Verification items for this drawing (mm, ordinates from the low corner). A direction names the side the tool comes from. Round coordinates to 2 decimals unless told otherwise and drop trailing zeros. Order: outer loops, then holes, each group sorted by start corner. A loop starts at its lowest first (then second) coordinate and runs counter-clockwise, first axis right, second up. Notation, with made-up numbers: (47, 22.25) -> (84, 22.25) arc R7 ccw to (84, 26.25) -> close; hole circle Ø3 at (-32, 67.5). An arc over 180 degrees is marked (long way). Put each result on its own line as item: value.
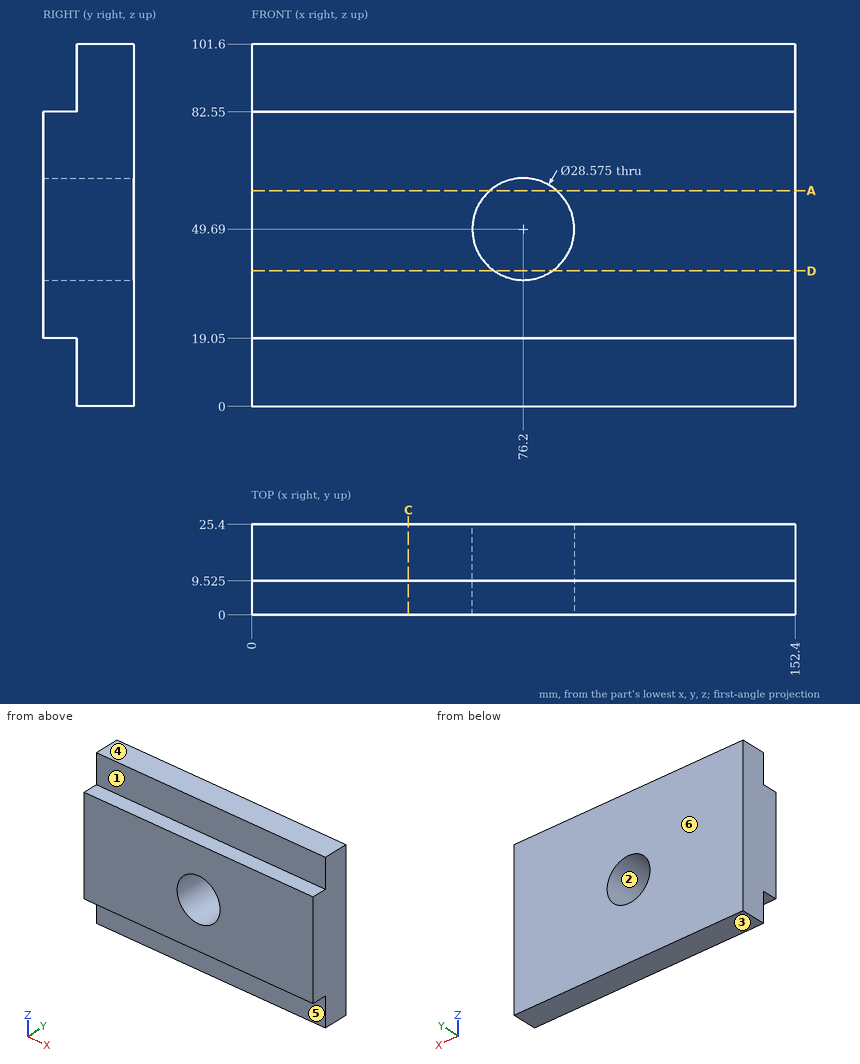
Item 1: Material ranges on L1, parallel to Z at x = 76.2, y = 10; L2, parallel to Z at x = 76.2, y = 5.75; L3, parallel to Y at x = 12.5, z = 93.5 (3 decimals), recorded low to high. Write a range as [from, to].
Check sheet entries:
L1: z = [0, 35.4], [63.98, 101.6]
L2: z = [19.05, 35.4], [63.98, 82.55]
L3: y = [9.525, 25.4]
Item 2: Section check D-D on z = 38. Record the boundary of the cut face in (x, y), then the cut area to 3 significant figures.
Check sheet entries:
outline: (0, 0) -> (67.99, 0) -> (67.99, 25.4) -> (0, 25.4) -> close; (84.41, 0) -> (152.4, 0) -> (152.4, 25.4) -> (84.41, 25.4) -> close
area: 3,450 mm^2
Item 3: Tool access check on the marked faces 5 and 6. Record the directions out of +Z, -Z, +X, -X, +Y, -Y that give a thin tool (end or side, any length) a straight path to the whole face; none if there is none.
Check sheet entries:
face 5: -Z, +X, -X, -Y
face 6: +Z, -Z, +X, -X, +Y
Item 4: Section check A-A on z = 60.5. Record the boundary of the cut face in (x, y).
Check sheet entries:
outline: (0, 0) -> (66.86, 0) -> (66.86, 25.4) -> (0, 25.4) -> close; (85.54, 0) -> (152.4, 0) -> (152.4, 25.4) -> (85.54, 25.4) -> close
Item 5: Gauge pin test, flat ends, axial feed: pin 1 Ø7.5 at (x, y) = (46, 4.5) entering from -Z; pin 2 Ø9.5 at (x, z) = (114, 5.5) entering from -Y (3 decimals); pin 3 Ø7.5 at (x, y) = (108, 5.5) entering from +Z. Record the tip position at first contact, or that the pin passes through.
Check sheet entries:
pin 1: stops at z = 19.05
pin 2: stops at y = 9.525
pin 3: stops at z = 82.55
Item 6: Release check for a two-part mould opening along Z. For the marked faces 1, 2, 3 and 4 record: +Z half, -Z half, draft (parallel to the pull), parting line (faces both ways), or undercut.
Check sheet entries:
face 1: draft
face 2: undercut
face 3: -Z half
face 4: +Z half
Item 7: Section check C-C on x = 44. Record the boundary of the cut face in (y, z) (3 decimals).
Check sheet entries:
outline: (0, 19.05) -> (9.525, 19.05) -> (9.525, 0) -> (25.4, 0) -> (25.4, 101.6) -> (9.525, 101.6) -> (9.525, 82.55) -> (0, 82.55) -> close
